Model file for the job. Use its own axes, mm. A direction names the side the tool comes from. Round coordinates to 2 decimals unless told otherwise and drop trailing zeros. Order: outer loops, then holes, each group sorted by start corner. A loop starts at its lowest first (then second) coordinate and runs counter-clockwise, first axis right, second up. Notation, with made-up numbers: (-2, 82.5) - (13, 82.5) arc R23 ccw to (13, 110.5) - close; hole circle Ø4 at (61.5, -23.75). An arc over 180 degrees is marked (long way). Write item = value, one per line.
```python
from build123d import *

# Parameters (mm, degrees)
SKETCH_1_R          = 37.5
EXTRUDE_3_DEPTH     = 14
SKETCH_2_R          = 39.5
SKETCH_2_R_2        = 37.5
EXTRUDE_4_DEPTH     = 2
EXTRUDE_START       = -2
SKETCH_3_R          = 39.5
SKETCH_3_R_2        = 37.5
EXTRUDE_5_DEPTH     = 2
SKETCH_4_R          = 39.5
CUT_EXTRUDE_1_DEPTH = 2
SKETCH_5_R          = 1.5
CUT_EXTRUDE_3_DEPTH = 58.135803136
SKETCH_6_W          = 40
SKETCH_6_H          = 40
EXTRUDE_6_DEPTH     = 10
SKETCH_7_W          = 15
SKETCH_7_H          = 7
EXTRUDE_7_DEPTH     = 30
SKETCH_8_W          = 3
SKETCH_8_H          = 14.2
EXTRUDE_9_DEPTH     = 10
EXTRUDE_10_DEPTH    = 20
SKETCH_10_R         = 1.5
CUT_EXTRUDE_4_DEPTH = 20
FILLET_1_R          = 3
EXTRUDE_START_2     = 6.5
SKETCH_11_W         = 22
SKETCH_11_H         = 14.2
SKETCH_11_R         = 1.5
EXTRUDE_11_DEPTH    = 6.5
CHAMFER_1_SIZE      = 6.5
SKETCH_12_R         = 3
CUT_EXTRUDE_5_DEPTH = 4
SKETCH_13_R         = 2.25
CUT_EXTRUDE_6_DEPTH = 10
SKETCH_15_R         = 2.25
CUT_EXTRUDE_7_DEPTH = 10


with BuildPart() as part:
    # 草图1 → 凸台-拉伸3 (new body)
    with BuildSketch(Plane.XY):
        Circle(SKETCH_1_R)
    extrude(amount=EXTRUDE_3_DEPTH)

    # 草图2 → 凸台-拉伸4 (add)
    with BuildSketch(Plane(origin=(0, 0, 0), x_dir=(-1, 0, 0), z_dir=(0, 0, -1))):
        Circle(SKETCH_2_R)
        Circle(SKETCH_2_R_2, mode=Mode.SUBTRACT)
    extrude(amount=-EXTRUDE_4_DEPTH)

    # 草图3 → 凸台-拉伸5 (add)
    with BuildSketch(Plane.XY.offset(14).offset(EXTRUDE_START)):
        with Locations(Location((0, 0, 0), (0, 0, 180))):
            Circle(SKETCH_3_R)
        with Locations(Location((0, 0, 0), (0, 0, 180))):
            Circle(SKETCH_3_R_2, mode=Mode.SUBTRACT)
    extrude(amount=EXTRUDE_5_DEPTH)

    # 草图4 → 切除-拉伸1 (cut)
    with BuildSketch(Plane(origin=(0, 0, 0), x_dir=(-1, 0, 0), z_dir=(0, 0, -1))):
        with Locations(Location((0, 0, 0), (0, 0, 180))):
            Circle(SKETCH_4_R)
    extrude(amount=-CUT_EXTRUDE_1_DEPTH, mode=Mode.SUBTRACT)

    # 草图5 → 切除-拉伸3 (cut, through all)
    with BuildSketch(Plane(origin=(0, 0, 2), x_dir=(-1, 0, 0), z_dir=(0, 0, -1))):
        with Locations((0, -33)):
            Circle(SKETCH_5_R)
        with Locations((-28.578838325, 16.5)):
            Circle(SKETCH_5_R)
        with Locations((28.578838325, 16.5)):
            Circle(SKETCH_5_R)
    extrude(amount=-CUT_EXTRUDE_3_DEPTH, mode=Mode.SUBTRACT)

    # 草图6 → 凸台-拉伸6 (add)
    with BuildSketch(Plane(origin=(0, 0, 2), x_dir=(-1, 0, 0), z_dir=(0, 0, -1))):
        Rectangle(SKETCH_6_W, SKETCH_6_H)
    extrude(amount=EXTRUDE_6_DEPTH)

    # 草图7 → 凸台-拉伸7 (add)
    with BuildSketch(Plane(origin=(0, 0, 2), x_dir=(-1, 0, 0), z_dir=(0, 0, -1))):
        with Locations((-2.5, -23.5)):
            Rectangle(SKETCH_7_W, SKETCH_7_H)
        with Locations((-2.5, 23.5)):
            Rectangle(SKETCH_7_W, SKETCH_7_H)
    extrude(amount=EXTRUDE_7_DEPTH)

    # 草图8 → 凸台-拉伸9 (add)
    with BuildSketch(Plane(origin=(0, 0, -8), x_dir=(-1, 0, 0), z_dir=(0, 0, -1))):
        with Locations((21.5, 9.9)):
            Rectangle(SKETCH_8_W, SKETCH_8_H)
        with Locations((18.5, 9.9)):
            Rectangle(SKETCH_8_W, SKETCH_8_H)
    extrude(amount=-EXTRUDE_9_DEPTH)

    # 草图9 → 凸台-拉伸10 (add)
    with BuildSketch(Plane(origin=(0, 0, -8), x_dir=(-1, 0, 0), z_dir=(0, 0, -1))):
        Polygon((23, 17), (17, 17), (17, 2.9), (23, 2.8), align=None)
    extrude(amount=EXTRUDE_10_DEPTH)

    # 草图10 → 切除-拉伸4 (cut)
    with BuildSketch(Plane.ZY.offset(23)):
        with Locations((-17.84, 9.9)):
            Circle(SKETCH_10_R)
    extrude(amount=-CUT_EXTRUDE_4_DEPTH, mode=Mode.SUBTRACT)

    # 圆角1
    fillet_1_edges = [part.edges().sort_by_distance(p)[0] for p in [
        (-20, -20, -3),
        (-20, 20, -3),
        (20, 20, -3),
        (20, -20, -3),
    ]]
    fillet(fillet_1_edges, radius=FILLET_1_R - 0.0001)  # a hair under: the kernel refuses the full size

    # 草图11 → 凸台-拉伸11 (add)
    with BuildSketch(Plane.ZY.offset(23).offset(EXTRUDE_START_2)):
        with Locations((-17, 9.9)):
            Rectangle(SKETCH_11_W, SKETCH_11_H)
        with Locations((-17.84, 9.9)):
            Circle(SKETCH_11_R, mode=Mode.SUBTRACT)
    extrude(amount=-EXTRUDE_11_DEPTH)

    # 倒角1
    chamfer_1_edges = [part.edges().sort_by_distance(p)[0] for p in [
        (-29.5, 9.9, -6),
    ]]
    chamfer(chamfer_1_edges, length=CHAMFER_1_SIZE - 0.0001)  # a hair under: the kernel refuses the full size

    # 草图12 → 切除-拉伸5 (cut)
    with BuildSketch(Plane(origin=(-17, 0, 0), x_dir=(0, 0, -1), z_dir=(1, 0, 0))):
        with Locations((17.84, 9.9)):
            Circle(SKETCH_12_R)
    extrude(amount=-CUT_EXTRUDE_5_DEPTH, mode=Mode.SUBTRACT)

    # 草图13 → 切除-拉伸6 (cut)
    with BuildSketch(Plane(origin=(10, 0, 0), x_dir=(0, 0, -1), z_dir=(1, 0, 0))):
        with Locations((23.1, -24)):
            Circle(SKETCH_13_R)
        with Locations((13.1, -24)):
            Circle(SKETCH_13_R)
    extrude(amount=-CUT_EXTRUDE_6_DEPTH, mode=Mode.SUBTRACT)

    # 草图15 → 切除-拉伸7 (cut)
    with BuildSketch(Plane(origin=(10, 0, 0), x_dir=(0, 0, -1), z_dir=(1, 0, 0))):
        with Locations((23.1, 24)):
            Circle(SKETCH_15_R)
        with Locations((13.1, 24)):
            Circle(SKETCH_15_R)
    extrude(amount=-CUT_EXTRUDE_7_DEPTH, mode=Mode.SUBTRACT)


solid = part.part
```
1) Wall check: line 1 along Y through (x, z) = (4.25, -13.1); line 2 along Y through (x, z) = (0, 5.5); line 3 along Z through (x, y) = (-24.5, -16). Give the ranges that are in metal, low to high.
Conclusion:
line_1 = -27 to -26.25, -21.75 to -20, 20 to 21.75, 26.25 to 27
line_2 = -37.5 to -34.5, -31.5 to 37.5
line_3 = 2 to 14
2) Mould opens along Z. For faces 1 (the face through (0, -24, -23)), 2 (the face through (3, 20, -18)), 3 (the face through (-35, 14, 12)), 4 (the face through (5.07, 21.804, -12.612)) say: +Z half, -Z half, draft (parallel to the pull), parting line (faces both ways), or undercut.
Conclusion:
face_1 = undercut
face_2 = draft
face_3 = -Z half
face_4 = undercut
3) Cut at D-D (y = 30). Write the cut outline in (x, z).
Conclusion:
outline = (-25.7, 12) - (-22.5, 12) - (-22.5, 2) - (22.5, 2) - (22.5, 12) - (25.7, 12) - (25.7, 14) - (-25.7, 14) - close
4) Flat gauge pins, fed straight in: pin 1 Ø3 at (y, z) = (10, -17.5) entering from +X; pin 2 Ø5 at (y, z) = (-25, -22.5) entering from +X; pin 3 Ø2 at (x, z) = (12, -1.5) entering from -Y. Where does each tip first touch, or does it go through?
Conclusion:
pin_1 = -21
pin_2 = 10
pin_3 = -20
5) Cut at A-A (z = -17.84). Write the cut outline in (x, y), and give its area (3 significant figures).
Conclusion:
outline = (-29.5, 2.8) - (-23, 2.8) - (-17, 2.9) - (-17, 6.9) - (-21, 6.9) - (-21, 8.4) - (-29.5, 8.4) - close; (-29.5, 11.4) - (-21, 11.4) - (-21, 12.9) - (-17, 12.9) - (-17, 17) - (-29.5, 17) - close; (-5, -27) - (10, -27) - (10, -20) - (-5, -20) - close; (-5, 20) - (10, 20) - (10, 27) - (-5, 27) - close
area = 338 mm^2
6) 3-axis set-ups, long thin cutter, end or side, ignore diameter. For faces 5 (the face through (0, 24, -23)), 6 (the face through (3, -20, -18)), 7 (the face through (19.14, 19.1, -3.07)), 8 (the face through (-19.14, 19.1, -3.07)): which of +Z, -Z, +X, -X, +Y, -Y reach the whole face in a straight line?
Conclusion:
face_5 = +X
face_6 = -Z, +X, -X
face_7 = -Z, +X, +Y
face_8 = -Z, -X, +Y
7) Cut at C-C (x = 12). Write the cut outline in (y, z).
Conclusion:
outline = (-37.63, 12) - (-35.53, 12) - (-35.53, 2) - (-20, 2) - (-20, -8) - (20, -8) - (20, 2) - (35.53, 2) - (35.53, 12) - (37.63, 12) - (37.63, 14) - (-37.63, 14) - close
